from build123d import *

# Parameters (mm, degrees)
SKETCH_1_R                  = 2
EXTRUDE_1_DEPTH             = 8
HOLE_WIZARD_M41_D           = 3.3
HOLE_WIZARD_M41_DEPTH       = 14.999
HOLE_WIZARD_M41_CSINK_D     = 4.05
HOLE_WIZARD_M41_CSINK_ANGLE = 90
HOLE_WIZARD_M41_TIP         = 0.991420021


with BuildPart() as part:
    # Эскиз1 → Бобышка-Вытянуть1 (new body)
    with BuildSketch(Plane.XY):
        with BuildLine():
            Line((-4, 15), (-4, 0))
            ThreePointArc((-4, 0), (0, -4), (4, 0))
            Line((4, 0), (4, 15))
            Line((4, 15), (-4, 15))
        make_face()
        Circle(SKETCH_1_R, mode=Mode.SUBTRACT)
    extrude(amount=EXTRUDE_1_DEPTH)

    # Отверстие обработанное метчиком M41
    with Locations(Plane(origin=(0, 15, 0), x_dir=(1, 0, 0), z_dir=(0, 1, 0))):
        with Locations((0, -4)):
            CounterSinkHole(HOLE_WIZARD_M41_D / 2, HOLE_WIZARD_M41_CSINK_D / 2, depth=HOLE_WIZARD_M41_DEPTH, counter_sink_angle=HOLE_WIZARD_M41_CSINK_ANGLE)
            with Locations((0, 0, -(HOLE_WIZARD_M41_DEPTH + HOLE_WIZARD_M41_TIP / 2))):  # 118° drill point
                Cone(0, HOLE_WIZARD_M41_D / 2, HOLE_WIZARD_M41_TIP, mode=Mode.SUBTRACT)


solid = part.part
Here's how the part is built. I have some questions about the finished solid (model axes, mm). A direction names the side the tool comes from. Round coordinates to 2 decimals unless told otherwise and drop trailing zeros. Write each loop counter-clockwise with the first axis right and the second up, starting at its lowest first coordinate (ties: lowest second). Pieces come first, ordered by that corner, then holes. Notation, with made-up numbers: (-21, 62) -> (-9, 62) arc R31 cw to (-9, 87) -> close; hole circle Ø5 at (3, 4.5). An arc over 180 degrees is marked (long way). One line per item, written item: value.
1) I'm going to push a flat-ended pin straight in: pin 1 Ø2 at (x, z) = (0, 4) entering from +Y. Where does the tip first touch, or does it pass through?
Filled sheet:
pin 1: stops at y = -1.73
2) If I drill on line 1 (Z direction, x = 0, y = 9); line 2 (Y direction, x = 0, z = 4.5); line 3 (Y direction, x = -0.5, z = 0.5), over which ranges is the centre line in solid material (lowest first)? Write a range as [from, to].
Filled sheet:
line 1: z = [0, 2.35], [5.65, 8]
line 2: y = [-4, -2]
line 3: y = [-3.97, -1.94], [1.94, 15]
3) Suppose I cut it at B-B on z = 4. List the corners of the cut face in (x, y) for me (3 decimals).
Filled sheet:
outline: (-4, 0) arc R4 ccw to (4, 0) -> (4, 15) -> (2.025, 15) -> (1.65, 14.625) -> (1.65, 1.13) arc R2 cw (long way) to (-1.65, 1.13) -> (-1.65, 14.625) -> (-2.025, 15) -> (-4, 15) -> close
4) Suppose I cut it at D-D on z = 1.5. List the corners of the cut face in (x, y) for me.
Filled sheet:
outline: (-4, 0) arc R4 ccw to (4, 0) -> (4, 15) -> (-4, 15) -> close; hole circle Ø4 at (0, 0)
5) Suppose I cut it at C-C on y = 8.5. List the corners of the cut face in (x, z) for me, plus the area to 3 significant figures.
Filled sheet:
outline: (-4, 0) -> (4, 0) -> (4, 8) -> (-4, 8) -> close; hole circle Ø3.3 at (0, 4)
area: 55.4 mm2
6) For faces 5 (the face through (2, 15, 3)), 6 (the face through (1.65, 7.78, 3.93)), which set-ups out of +Z, -Z, +X, -X, +Y, -Y let a thin tool reach every point of the face, with its end or its side?
Filled sheet:
face 5: +Z, -Z, +X, -X, +Y
face 6: +Y
7) Suppose I cut it at A-A on x = 0. List the corners of the cut face in (y, z) for me (3 decimals), plus the area to 3 significant figures.
Filled sheet:
outline: (-4, 0) -> (-2, 0) -> (-2, 8) -> (-4, 8) -> close; (2, 0) -> (15, 0) -> (15, 1.975) -> (14.625, 2.35) -> (2, 2.35) -> close; (2, 5.65) -> (14.625, 5.65) -> (15, 6.025) -> (15, 8) -> (2, 8) -> close
area: 77.0 mm2
8) We'd pull the mould along X, two halves only. Please class faces 1 (the face through (4, 7, 4)), 2 (the face through (0, 6, 8)), 3 (the face through (-4, 8, 4)), 4 (the face through (0, -2, 4)): released by +X, released by -X, zero draft, split by the parting line, or undercut.
Filled sheet:
face 1: released by +X
face 2: zero draft
face 3: released by -X
face 4: undercut
